from build123d import *

# Parameters (mm, degrees)
SKETCH1_W           = 200
SKETCH1_H           = 200
BOSS_EXTRUDE1_DEPTH = 200
SKETCH3_W           = 200
SKETCH3_H           = 12.5
BOSS_EXTRUDE2_DEPTH = 20
SKETCH4_W           = 220
SKETCH4_H           = 12.5
BOSS_EXTRUDE3_DEPTH = 20
SKETCH5_W           = 220
SKETCH5_H           = 12.5
BOSS_EXTRUDE4_DEPTH = 20
SKETCH6_W           = 240
SKETCH6_H           = 12.5
BOSS_EXTRUDE5_DEPTH = 20
FILLET1_R           = 50
FILLET2_R           = 5


with BuildPart() as part:
    # Sketch1 → Boss-Extrude1 (new body)
    with BuildSketch(Plane(origin=(0, 0, 0), x_dir=(1, 0, 0), z_dir=(0, 1, 0))):
        with Locations((100, 100)):
            Rectangle(SKETCH1_W, SKETCH1_H)
    extrude(amount=BOSS_EXTRUDE1_DEPTH)

    # Sketch3 → Boss-Extrude2 (add)
    with BuildSketch(Plane.XY):
        with Locations((100, 6.25)):
            Rectangle(SKETCH3_W, SKETCH3_H)
    extrude(amount=BOSS_EXTRUDE2_DEPTH)

    # Sketch4 → Boss-Extrude3 (add)
    with BuildSketch(Plane(origin=(200, 0, 0), x_dir=(0, 0, -1), z_dir=(1, 0, 0))):
        with Locations((90, 6.25)):
            Rectangle(SKETCH4_W, SKETCH4_H)
    extrude(amount=BOSS_EXTRUDE3_DEPTH)

    # Sketch5 → Boss-Extrude4 (add)
    with BuildSketch(Plane(origin=(0, 0, -200), x_dir=(-1, 0, 0), z_dir=(0, 0, -1))):
        with Locations((-110, 6.25)):
            Rectangle(SKETCH5_W, SKETCH5_H)
    extrude(amount=BOSS_EXTRUDE4_DEPTH)

    # Sketch6 → Boss-Extrude5 (add)
    with BuildSketch(Plane.ZY):
        with Locations((-100, 6.25)):
            Rectangle(SKETCH6_W, SKETCH6_H)
    extrude(amount=BOSS_EXTRUDE5_DEPTH)

    # Fillet1
    fillet1_edges = [part.edges().sort_by_distance(p)[0] for p in [
        (220, 6.25, 20),
        (220, 6.25, -220),
        (-20, 6.25, -220),
        (-20, 6.25, 20),
    ]]
    fillet(fillet1_edges, radius=FILLET1_R)

    # Fillet2
    fillet2_edges = [part.edges().sort_by_distance(p)[0] for p in [
        (200, 200, -100),
        (100, 200, -200),
        (0, 200, -100),
        (100, 200, 0),
        (0, 106.25, -200),
        (200, 106.25, -200),
        (200, 106.25, 0),
        (0, 106.25, 0),
    ]]
    fillet(fillet2_edges, radius=FILLET2_R)


solid = part.part
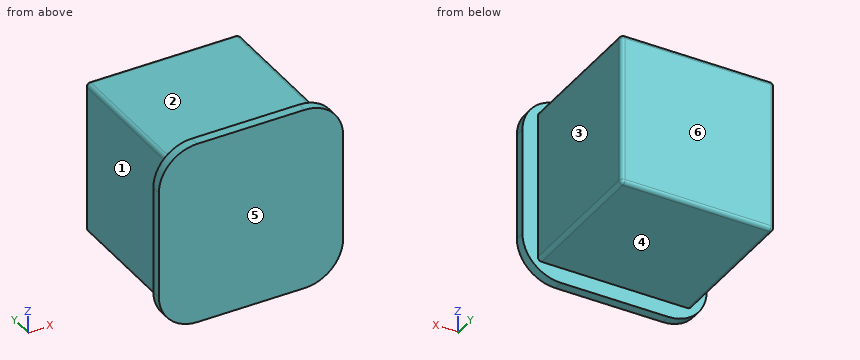
Here's how the part is built. I have some questions about the finished solid (model axes, mm). Face numbers are marked on the shaded views. A direction names the side the tool comes from. Give positions to 0.01 mm unless a question says otherwise; leave off trailing zeros. Loops run counter-clockwise (first coordinate to the right, second up) from the corner with the lowest first, then second, coordinate; pieces in that order, holes last. Notation, with made-up numbers: (62.25, 48) -> (88.25, 48) arc R23 ccw to (88.25, 66) -> close; hole circle Ø7 at (85, 35.5). An arc over 180 degrees is marked (long way). Answer as a JSON object with one key per item and string values. Group by question number.
Item 1: Imagine slicing it at B-B on y = 110. Write out the boundary of the cut face in (x, z).
Item 2: On a 3-axis mill with a long thin cutter (end or side, diameter ignored), from which of +Z, -Z, +X, -X, +Y, -Y can I reach the whole of each face in a straight line? I mean the marked faces 1, 2 and 3. Say none if no direction works.
Item 3: Imagine slicing it at C-C on z = -58.5. Write out the boundary of the cut face in (x, y), then the cut area to 3 significant figures.
Item 4: Imagine slicing it at A-A on x = 136. Write out the boundary of the cut face in (y, z), then the cut area to 3 significant figures.
Item 5: I need wall thicknesses on L1, parallel to X at y = 102, z = -155.5; L2, parallel to Z at x = 130, y = 89.5; L3, parallel to Y at x = 70, z = -207.5. Which ranges of each line are inside material? Lowest first, please.
Item 6: Will these pins go through, and if not, where does the flat tip stop? pin 1 (2 mm diameter, centred on x = 141, y = 43, fed in from -Z); pin 2 (5 mm diameter, centred on x = 132, y = 178.5, fed in from +Z); pin 3 (2 mm diameter, centred on y = 68.5, z = -73, fed in from +X).
Item 7: Thinking about a two-plate mould opening in Y: for the marked faces 4, 5 and 6, which applies, pulls with the +Y half, pulls with the -Y half, needs draft (parallel to the pull), parting line crosses it, or undercut?
Answer list:
{
 "1": {"outline": "(0, -195) arc R5 ccw to (5, -200) -> (195, -200) arc R5 ccw to (200, -195) -> (200, -5) arc R5 ccw to (195, 0) -> (5, 0) arc R5 ccw to (0, -5) -> close"},
 "2": {"face 1": "+Z, -Z, -X, +Y", "face 2": "+Z, +X, -X, +Y", "face 3": "+Z, -Z, +X, +Y"},
 "3": {"outline": "(-20, 0) -> (220, 0) -> (220, 12.5) -> (200, 12.5) -> (200, 195) arc R5 ccw to (195, 200) -> (5, 200) arc R5 ccw to (0, 195) -> (0, 12.5) -> (-20, 12.5) -> close", "area": "40,500 mm2"},
 "4": {"outline": "(0, -220) -> (12.5, -220) -> (12.5, -200) -> (195, -200) arc R5 ccw to (200, -195) -> (200, -5) arc R5 ccw to (195, 0) -> (12.5, 0) -> (12.5, 20) -> (0, 20) -> close", "area": "40,500 mm2"},
 "5": {"L1": "x = 0 to 200", "L2": "z = -200 to 0", "L3": "y = 0 to 12.5"},
 "6": {"pin 1": "stops at z = -200", "pin 2": "stops at z = 0", "pin 3": "stops at x = 200"},
 "7": {"face 4": "needs draft", "face 5": "pulls with the -Y half", "face 6": "pulls with the +Y half"}
}
